Could you check a few things on this drawing? It's one solid part, dimensions in mm from its lowest x, y, z. A direction names the side the tool comes from. Give positions to 0.01 mm unless a question says otherwise; leave off trailing zeros. Loops run counter-clockwise (first coordinate to the right, second up) from the corner with the lowest first, then second, coordinate; pieces in that order, holes last. Notation, with made-up numbers: (-12, 71.5) -> (22, 71.5) arc R33 cw to (22, 105.5) -> close; hole circle Ø3 at (-7, 76.25). An arc over 180 degrees is marked (long way). One line per question, with ' | ' between items.
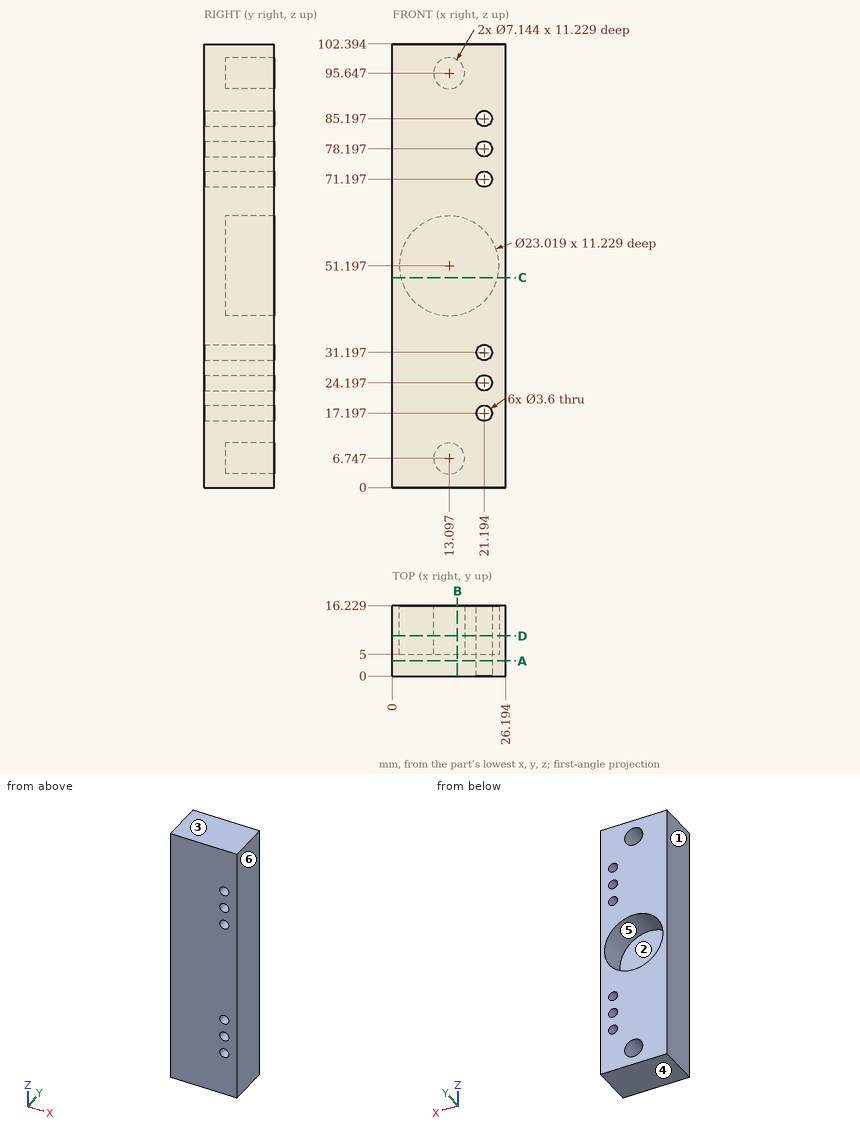
Q1. On a 3-axis mill with a long thin cutter (end or side, diameter ignored), from which of +Z, -Z, +X, -X, +Y, -Y can I reach the whole of each face in a straight line? I mean the marked faces 1 and 2. Say none if no direction works.
Entries:
face 1: +Z, -Z, -X, +Y, -Y | face 2: +Y
Q2. If we section it at A-A (y = 3.5): Write out the boundary of the cut face in (x, z).
Entries:
outline: (0, 0) -> (26.19, 0) -> (26.19, 102.39) -> (0, 102.39) -> close; hole circle Ø3.6 at (21.19, 17.2); hole circle Ø3.6 at (21.19, 24.2); hole circle Ø3.6 at (21.19, 31.2); hole circle Ø3.6 at (21.19, 71.2); hole circle Ø3.6 at (21.19, 78.2); hole circle Ø3.6 at (21.19, 85.2)
Q3. If I drill on probe 1 along Z at (x, y) = (11, 13.25) (1 decimal); probe 2 along X at (y, z) = (9, 31) (1 decimal); probe 3 along Z at (x, y) = (15.75, 5.75) (1 decimal), over which ranges is the centre line in solid material (lowest first)? Write a range as from..to.
Entries:
probe 1: 0..3.9, 9.6..39.9, 62.5..92.8, 98.5..102.4 | probe 2: 0..19.4, 23..26.2 | probe 3: 0..4.4, 9.1..40, 62.4..93.3, 98..102.4
Q4. If we section it at C-C (z = 48.5): Write out the boundary of the cut face in (x, y).
Entries:
outline: (0, 0) -> (26.19, 0) -> (26.19, 16.23) -> (24.29, 16.23) -> (24.29, 5) -> (1.91, 5) -> (1.91, 16.23) -> (0, 16.23) -> close
Q5. If we section it at D-D (y = 9.25): State how many separate pieces and enclosed holes the cut face has, plus the area to 3 significant figures.
Entries:
separate pieces: 1 | enclosed holes: 9 | area: 2,120 mm²
Q6. For pin 1 Ø6.5 at (x, z) = (13.1, 95.65) entering from +Y; pin 2 Ø2 at (x, z) = (21.19, 71.2) entering from +Y, each with a flat end and sliding along its axis, tell me the tip position at first contact or that it passes through.
Entries:
pin 1: y = 5 | pin 2: through
Q7. If we section it at B-B (x = 15): Write out the boundary of the cut face in (y, z).
Entries:
outline: (0, 0) -> (16.23, 0) -> (16.23, 3.72) -> (5, 3.72) -> (5, 9.77) -> (16.23, 9.77) -> (16.23, 39.85) -> (5, 39.85) -> (5, 62.55) -> (16.23, 62.55) -> (16.23, 92.62) -> (5, 92.62) -> (5, 98.67) -> (16.23, 98.67) -> (16.23, 102.39) -> (0, 102.39) -> close
Q8. If we mould it in two halves opening along Z, with no side actions, what happens to the marked faces 3, 4, 5 and 6? For each: pulls with the +Z half, pulls with the -Z half, needs draft (parallel to the pull), parting line crosses it, or undercut.
Entries:
face 3: pulls with the +Z half | face 4: pulls with the -Z half | face 5: undercut | face 6: needs draft
